```python
from build123d import *

# Parameters (mm, degrees)
ESQUISSE2_W             = 230
ESQUISSE2_H             = 80
BOSS_EXTRU_1_DEPTH      = 3
ESQUISSE3_W             = 28
ESQUISSE3_H             = 3
ESQUISSE3_W_2           = 19
BOSS_EXTRU_2_DEPTH      = 3
ESQUISSE5_W             = 5.353052469
ESQUISSE5_H             = 20
ESQUISSE5_W_2           = 7.144707487
BOSS_EXTRU_3_DEPTH      = 3
ESQUISSE7_W             = 4.903552449
ESQUISSE7_H             = 20
ENL_V_MAT_EXTRU_2_DEPTH = 10
ESQUISSE8_W             = 2.353052469
ESQUISSE8_H             = 20
ENL_V_MAT_EXTRU_3_DEPTH = 10
ESQUISSE9_R             = 5
ENL_V_MAT_EXTRU_4_DEPTH = 10


with BuildPart() as part:
    # Esquisse2 → Boss.-Extru.1 (new body)
    with BuildSketch(Plane.XY):
        with Locations((115, 40)):
            Rectangle(ESQUISSE2_W, ESQUISSE2_H)
    extrude(amount=BOSS_EXTRU_1_DEPTH)

    # Esquisse3 → Boss.-Extru.2 (add)
    with BuildSketch(Plane(origin=(0, 0, 0), x_dir=(-1, 0, 0), z_dir=(0, 0, -1))):
        with Locations((-45, 81.5)):
            Rectangle(ESQUISSE3_W, ESQUISSE3_H)
        with Locations((-105, 81.5)):
            Rectangle(ESQUISSE3_W, ESQUISSE3_H)
        with Locations((-165, 81.5)):
            Rectangle(ESQUISSE3_W, ESQUISSE3_H)
        with Locations((-220.5, 81.5)):
            Rectangle(ESQUISSE3_W_2, ESQUISSE3_H)
        with Locations((-45, -1.5)):
            Rectangle(ESQUISSE3_W, ESQUISSE3_H)
        with Locations((-105, -1.5)):
            Rectangle(ESQUISSE3_W, ESQUISSE3_H)
        with Locations((-165, -1.5)):
            Rectangle(ESQUISSE3_W, ESQUISSE3_H)
        with Locations((-220.5, -1.5)):
            Rectangle(ESQUISSE3_W_2, ESQUISSE3_H)
    extrude(amount=-BOSS_EXTRU_2_DEPTH)

    # Esquisse5 → Boss.-Extru.3 (add)
    with BuildSketch(Plane(origin=(0, 0, 0), x_dir=(-1, 0, 0), z_dir=(0, 0, -1))):
        with Locations((2.676526235, 10)):
            Rectangle(ESQUISSE5_W, ESQUISSE5_H)
        with Locations((3.572353744, 50)):
            Rectangle(ESQUISSE5_W_2, ESQUISSE5_H)
        with Locations((-232.676526235, 10)):
            Rectangle(ESQUISSE5_W, ESQUISSE5_H)
        with Locations((-233.572353744, 50)):
            Rectangle(ESQUISSE5_W_2, ESQUISSE5_H)
    extrude(amount=-BOSS_EXTRU_3_DEPTH)

    # Esquisse7 → Enl_v. mat.-Extru.2 (cut)
    with BuildSketch(Plane.XY.offset(3)):
        with Locations((235.451776225, 50)):
            Rectangle(ESQUISSE7_W, ESQUISSE7_H)
        with Locations((-5.451776224, 50)):
            Rectangle(ESQUISSE7_W, ESQUISSE7_H)
    extrude(amount=-ENL_V_MAT_EXTRU_2_DEPTH, mode=Mode.SUBTRACT)

    # Esquisse8 → Enl_v. mat.-Extru.3 (cut)
    with BuildSketch(Plane(origin=(0, 0, 0), x_dir=(-1, 0, 0), z_dir=(0, 0, -1))):
        with Locations((-234.176526235, 10)):
            Rectangle(ESQUISSE8_W, ESQUISSE8_H)
        with Locations((4.176526235, 10)):
            Rectangle(ESQUISSE8_W, ESQUISSE8_H)
    extrude(amount=-ENL_V_MAT_EXTRU_3_DEPTH, mode=Mode.SUBTRACT)

    # Esquisse9 → Enl_v. mat.-Extru.4 (cut)
    with BuildSketch(Plane.XY.offset(3)):
        with Locations((30, 40)):
            Circle(ESQUISSE9_R)
        with Locations((200, 40)):
            Circle(ESQUISSE9_R)
    extrude(amount=-ENL_V_MAT_EXTRU_4_DEPTH, mode=Mode.SUBTRACT)


solid = part.part
```
Here's how the part is built. I have some questions about the finished solid (model axes, mm). Give positions to 0.01 mm unless a question says otherwise; leave off trailing zeros. Write each loop counter-clockwise with the first axis right and the second up, starting at its lowest first coordinate (ties: lowest second). Pieces come first, ordered by that corner, then holes. Notation, with made-up numbers: (86, 67.5) -> (118, 67.5) arc R9 ccw to (118, 79.5) -> close; hole circle Ø1 at (12, 12.5). An arc over 180 degrees is marked (long way). Use one line per item in the form item = value.
1) If I drill on L1, parallel to X at y = 80.5, z = 0.35; L2, parallel to Y at x = 200, z = 1.75; L3, parallel to Y at x = 123.5, z = 1.7, over which ranges is the centre line in solid material (lowest first)? Write a range as [from, to].
Verdict:
L1 = [31, 59], [91, 119], [151, 179], [211, 230]
L2 = [0, 35], [45, 80]
L3 = [0, 80]
2) We'd pull the mould along Y, two halves only. Please class faces 1 (the face through (117, 41, 3)), 2 (the face through (26, 43, 2)): +Y half, -Y half, draft (parallel to the pull), parting line (faces both ways), or undercut.
Verdict:
face_1 = draft
face_2 = undercut
3) Suppose I cut it at B-B (z = 2.2). Give the number of separate pieces and of enclosed holes in the cut face, and give its area (3 significant figures).
Verdict:
separate_pieces = 1
enclosed_holes = 2
area = 19,100 mm2
4) I'm going to push flat-ended pins straight in: pin 1 (1.5 mm diameter, centred on y = 33, z = 1, fed in from -X); pin 2 (0.9 mm diameter, centred on y = -1.5, z = 1, fed in from -X); pin 3 (0.9 mm diameter, centred on x = 17, z = 2, fed in from -Y). Where does each tip first touch, or does it pass through?
Verdict:
pin_1 = 0
pin_2 = 31
pin_3 = 0
5) Suppose I cut it at A-A (x = 200). Please give me the cut outline in (y, z), and give its area (3 significant figures).
Verdict:
outline = (0, 0) -> (35, 0) -> (35, 3) -> (0, 3) -> close; (45, 0) -> (80, 0) -> (80, 3) -> (45, 3) -> close
area = 210 mm2
